Here's the drawing with two shaded views (mm, measured from the low corner). I have some questions. A direction names the side the tool comes from. Coordinates: 2 decimals unless noted, no trailing zeros. Write each loop counter-clockwise with the first axis right and the second up, starting at its lowest first coordinate (ties: lowest second). Pieces come first, ordered by that corner, then holes.
Item 1: For the marked faces 4, 5 and 6, which set-ups out of +Z, -Z, +X, -X, +Y, -Y let a thin tool reach every point of the face, with its end or its side?
Item 2: If we section it at C-C (x = 54): Please give me the cut outline in (y, z), then the cut area to 3 significant figures.
Item 3: I'm going to push flat-ended pins straight in: pin 1 Ø3 at (y, z) = (132.5, 30) entering from -X; pin 2 Ø2 at (x, y) = (45.5, 39) entering from -Z; pin 3 Ø20 at (x, y) = (43, 18.5) entering from +Z. Where does each tip first touch, or does it pass through?
Item 4: We'd pull the mould along X, two halves only. Please class the marked faces 1, 2 and 3: +X half, -X half, draft (parallel to the pull), parting line (faces both ways), or undercut.
Item 5: If we section it at B-B (z = 23.5): Please give me the cut outline in (x, y).
Item 6: If we section it at A-A (x = 129): Please give me the cut outline in (y, z).
Item 7: If we section it at D-D (y = 107.5): Please give me the cut outline in (x, z), then the cut area to 3 significant figures.
Item 8: If I drill on line 1 (Y direction, x = 114.5, z = 60); line 2 (Y direction, x = 134.5, z = 71.5); line 3 (X direction, y = 73.5, z = 16.5) (1 decimal), over which ranges is the centre line in solid material (lowest first)?
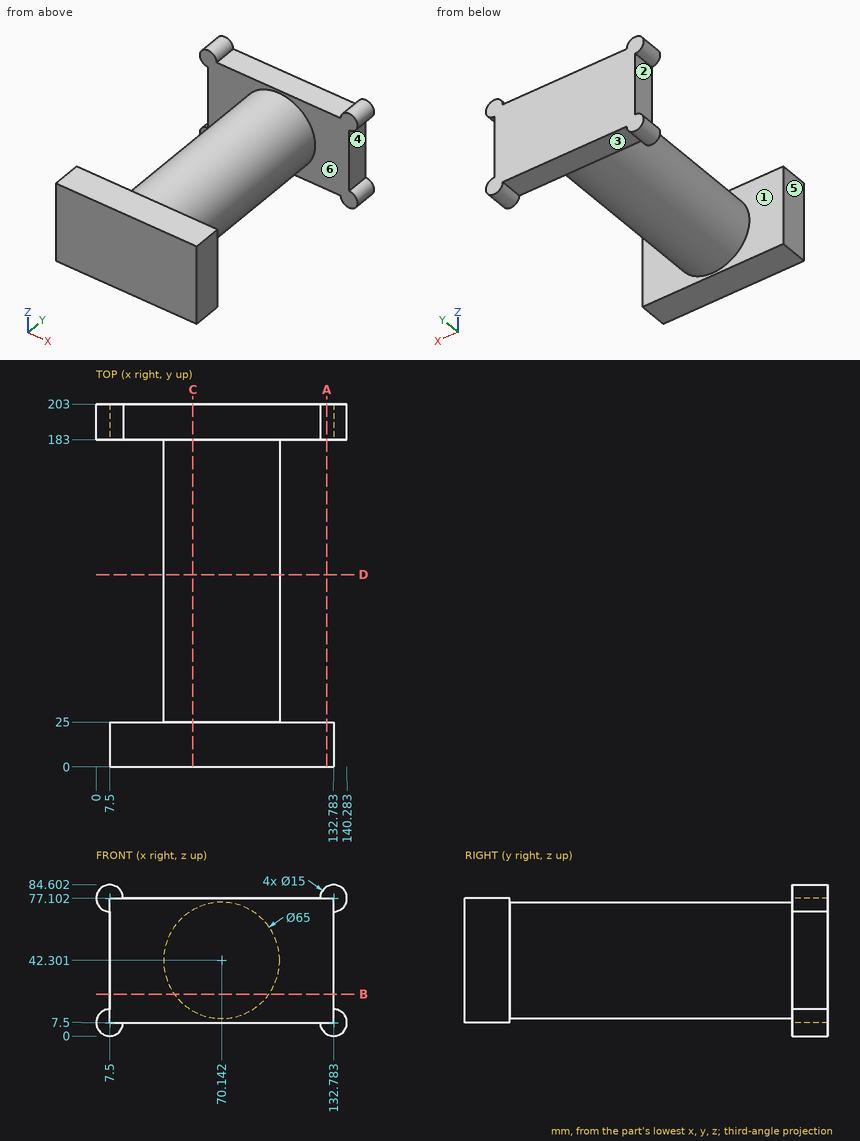
Answer list:
1. face 4: +X, +Y, -Y
1. face 5: +Z, -Z, -X, -Y
1. face 6: none
2. outline: (0, 7.5) - (25, 7.5) - (25, 14.09) - (183, 14.09) - (183, 7.5) - (203, 7.5) - (203, 77.1) - (183, 77.1) - (183, 70.51) - (25, 70.51) - (25, 77.1) - (0, 77.1) - close
2. area: 12,000 mm2
3. pin 1: stops at x = 39.49
3. pin 2: stops at z = 20
3. pin 3: stops at z = 77.1
4. face 1: draft
4. face 2: -X half
4. face 3: undercut
5. outline: (7.5, 0) - (132.78, 0) - (132.78, 25) - (96.65, 25) - (96.65, 183) - (132.78, 183) - (132.78, 203) - (7.5, 203) - (7.5, 183) - (43.63, 183) - (43.63, 25) - (7.5, 25) - close
6. outline: (0, 7.5) - (25, 7.5) - (25, 77.1) - (0, 77.1) - close; (183, 1.02) - (203, 1.02) - (203, 83.58) - (183, 83.58) - close
7. outline: circle Ø65 at (70.14, 42.3)
7. area: 3,320 mm2
8. line 1: y = 0 to 25, 183 to 203
8. line 2: y = 183 to 203
8. line 3: x = 50.4 to 89.9
